Source: CAD feature listing. Evaluate the final solid. Frame: model axes, mm. Face numbers are marked on the shaded views. A direction names the side the tool comes from. Coordinates: 2 decimals unless noted, no trailing zeros. Loops run counter-clockwise (first coordinate to the right, second up) from the corner with the lowest first, then second, coordinate; pieces in that order, holes last.
Item 1: Section query D-D, the plane z = 30.5. Return the cut outline in (x, y), then the cut area to 3 significant figures.
Item 2: Section query B-B, the plane y = -10.75. Return the cut outline in (x, z), then the cut area to 3 significant figures.
Item 3: Section query C-C, the plane x = -15. Return the cut outline in (y, z).
Item 4: Reachability of the marked faces 4 and 5 from +Z, -Z, +X, -X, +Y, -Y: full face, straight path, thin tool, end or side. Return the list, or none.
Item 5: Pin query (flat end, axial travel): pin 1 Ø2 at (x, z) = (15, 5) entering from +Y; pin 2 Ø12 at (x, y) = (2, -4) entering from +Z; pin 3 Ø2.5 at (x, z) = (-15, 35) entering from +Y. Return the tip coordinate at first contact, or that it passes through.
Item 6: Section query A-A, the plane z = 35. Return the cut outline in (x, y), then the cut area to 3 significant figures.
Item 7: Pull-direction query (X, two-part tool) for the marked faces 1, 2 and 3; classes: +X half, -X half, draft (parallel to the pull), parting line (faces both ways), or undercut.
Item 8: Line query: probe 1 along Z at (x, y) = (15, 12.85); probe 2 along X at (y, z) = (-4.5, 15.5); probe 3 along Y at (x, z) = (-17, 21). Output: solid intervals per line, ascending.
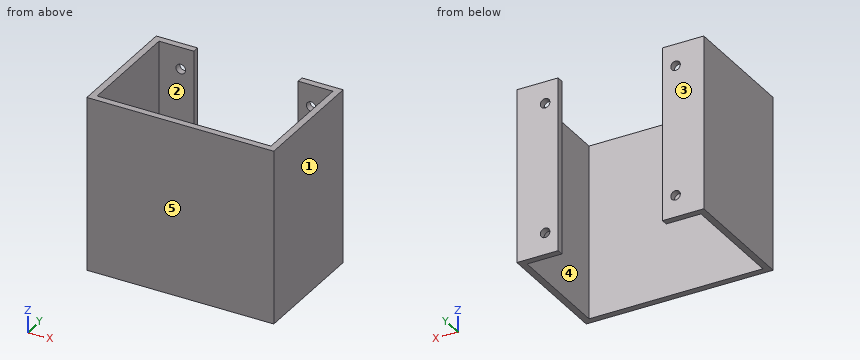
```python
from build123d import *

# Parameters (mm, degrees)
F1_DEPTH = 40
F2_R     = 1.1
F3_DEPTH = 1.5


with BuildPart() as f1:
    # F0 (on Top) → F1 (new body)
    with BuildSketch(Plane.XY):
        Polygon((-12, 14), (-21.5, 14), (-21.5, -14), (21.5, -14), (21.5, 14), (12, 14), (12, 12.5), (20, 12.5), (20, -12.5), (-20, -12.5), (-20, 12.5), (-12, 12.5), align=None)
    extrude(amount=F1_DEPTH)

    # F2 (on face) → F3 (cut, through all)
    with BuildSketch(Plane(origin=(0, 14, 0), x_dir=(-1, 0, 0), z_dir=(0, 1, 0))):
        with Locations((-15, 35)):
            Circle(F2_R)
        with Locations((15, 35)):
            Circle(F2_R)
        with Locations((-15, 5)):
            Circle(F2_R)
        with Locations((15, 5)):
            Circle(F2_R)
    extrude(amount=-F3_DEPTH, mode=Mode.SUBTRACT)


solid = f1.part
```
Verdict:
1. outline: (-21.5, -14) - (21.5, -14) - (21.5, 14) - (12, 14) - (12, 12.5) - (20, 12.5) - (20, -12.5) - (-20, -12.5) - (-20, 12.5) - (-12, 12.5) - (-12, 14) - (-21.5, 14) - close
1. area: 168 mm2
2. outline: (-21.5, 0) - (-20, 0) - (-20, 40) - (-21.5, 40) - close; (20, 0) - (21.5, 0) - (21.5, 40) - (20, 40) - close
2. area: 120 mm2
3. outline: (-14, 0) - (-12.5, 0) - (-12.5, 40) - (-14, 40) - close; (12.5, 0) - (14, 0) - (14, 3.9) - (12.5, 3.9) - close; (12.5, 6.1) - (14, 6.1) - (14, 33.9) - (12.5, 33.9) - close; (12.5, 36.1) - (14, 36.1) - (14, 40) - (12.5, 40) - close
4. face 4: +Z, -Z
4. face 5: +Z, -Z, +X, -X, -Y
5. pin 1: stops at y = -12.5
5. pin 2: passes through
5. pin 3: stops at y = 14
6. outline: (-21.5, -14) - (21.5, -14) - (21.5, 14) - (16.1, 14) - (16.1, 12.5) - (20, 12.5) - (20, -12.5) - (-20, -12.5) - (-20, 12.5) - (-16.1, 12.5) - (-16.1, 14) - (-21.5, 14) - close; (-13.9, 12.5) - (-12, 12.5) - (-12, 14) - (-13.9, 14) - close; (12, 12.5) - (13.9, 12.5) - (13.9, 14) - (12, 14) - close
6. area: 161 mm2
7. face 1: +X half
7. face 2: undercut
7. face 3: draft
8. probe 1: z = 0 to 3.9, 6.1 to 33.9, 36.1 to 40
8. probe 2: x = -21.5 to -20, 20 to 21.5
8. probe 3: y = -14 to -12.5, 12.5 to 14
